```python
from build123d import *

# Parameters (mm, degrees)
SKETCH_W     = 25.4
SKETCH_H     = 17.78
SKETCH_R     = 1.27
PAD_DEPTH    = 5
SKETCH001_R  = 4.65
PAD001_DEPTH = 11.25


with BuildPart() as part:
    # Sketch → Pad (new body)
    with BuildSketch(Plane.XY):
        Rectangle(SKETCH_W, SKETCH_H)
        with Locations((-10.16, 6.35)):
            Circle(SKETCH_R, mode=Mode.SUBTRACT)
        with Locations((10.16, 6.35)):
            Circle(SKETCH_R, mode=Mode.SUBTRACT)
        with Locations((10.16, -6.35)):
            Circle(SKETCH_R, mode=Mode.SUBTRACT)
        with Locations((-10.16, -6.35)):
            Circle(SKETCH_R, mode=Mode.SUBTRACT)
    extrude(amount=-PAD_DEPTH)

    # Sketch001 → Pad001 (join)
    with BuildSketch(Plane.XY):
        Circle(SKETCH001_R)
    extrude(amount=PAD001_DEPTH)


solid = part.part
```
Read the model definition and answer for the solid it produces. Units are mm, in the model's axes. A direction names the side the tool comes from. Give positions to 0.01 mm unless a question says otherwise; leave off trailing zeros. Order: outer loops, then holes, each group sorted by start corner. A loop starts at its lowest first (then second) coordinate and runs counter-clockwise, first axis right, second up. Notation, with made-up numbers: (33, -29.75) -> (50, -29.75) arc R22 ccw to (50, 7.25) -> close; hole circle Ø9 at (4, 42). An arc over 180 degrees is marked (long way). One line per item, written item: value. Start each with the question number.
(1) Flat-ended cylindrical pins translate along their axes: P1, Ø5, axis at x = -4, z = 9.5, coming from the -Y side; P2, Ø5, axis at x = -4.5, z = 8, coming from the -Y side; P3, Ø5, axis at y = -5, z = 8, coming from the -X side. Find the tip coordinate at first contact, or state that the pin passes through.
(2) A tool of negligible diameter and unlimited length cuts with its end or side. For faces 4 (the flat face through (0, 0, -5)), 5 (the cylindrical face through (2.5, 3.92, 5.55)), from which of +Z, -Z, +X, -X, +Y, -Y can it reach the whole face along a straight path? Write none if from no direction.
(3) The part is cut by section C-C (x = 10.16). Determine the outline of the cut face in (y, z).
(4) The part is cut by section B-B (y = -6.35). Determine the outline of the cut face in (x, z), and give its area (3 significant figures).
(5) The part is cut by section A-A (z = -0.5). Determine the outline of the cut face in (x, y), and give its area (3 significant figures).
(6) Straight lines are drawn through the part: L1, parallel to Y at x = -10.16, z = -1.4; L2, parallel to X at y = 7.5, z = -3; L3, parallel to Z at x = 8.75, y = 3.5. For each, find the intervals that lie inside material, in ascending order.
(7) The part is cut by section D-D (x = -1.25). Determine the outline of the cut face in (y, z).
(8) For a pull along Y with two mould halves and no side action, classify faces 1 (the flat face through (-12.7, 0, -2)), 2 (the cylindrical face through (9.224, 7.208, -2.465)), 3 (the flat face through (0, 8.89, -2)) as released by +Y, released by -Y, zero draft, split by the parting line, or undercut.
Taken from the geometry:
1. P1: y = -4.4
1. P2: y = -4.2
1. P3: x = -3.92
2. face 4: -Z, +X, -X, +Y, -Y
2. face 5: +Z
3. outline: (-8.89, -5) -> (-7.62, -5) -> (-7.62, 0) -> (-8.89, 0) -> close; (-5.08, -5) -> (5.08, -5) -> (5.08, 0) -> (-5.08, 0) -> close; (7.62, -5) -> (8.89, -5) -> (8.89, 0) -> (7.62, 0) -> close
4. outline: (-12.7, -5) -> (-11.43, -5) -> (-11.43, 0) -> (-12.7, 0) -> close; (-8.89, -5) -> (8.89, -5) -> (8.89, 0) -> (-8.89, 0) -> close; (11.43, -5) -> (12.7, -5) -> (12.7, 0) -> (11.43, 0) -> close
4. area: 102 mm^2
5. outline: (-12.7, -8.89) -> (12.7, -8.89) -> (12.7, 8.89) -> (-12.7, 8.89) -> close; hole circle Ø2.54 at (-10.16, -6.35); hole circle Ø2.54 at (-10.16, 6.35); hole circle Ø2.54 at (10.16, -6.35); hole circle Ø2.54 at (10.16, 6.35)
5. area: 431 mm^2
6. L1: -8.89 to -7.62, -5.08 to 5.08, 7.62 to 8.89
6. L2: -12.7 to -10.7, -9.62 to 9.62, 10.7 to 12.7
6. L3: -5 to 0
7. outline: (-8.89, -5) -> (8.89, -5) -> (8.89, 0) -> (4.48, 0) -> (4.48, 11.25) -> (-4.48, 11.25) -> (-4.48, 0) -> (-8.89, 0) -> close
8. face 1: zero draft
8. face 2: undercut
8. face 3: released by +Y
